```python
from build123d import *

# Parameters (mm, degrees)
F0_R      = 15.5
F1_DEPTH  = 75
F4_R      = 25.113735
F5_DEPTH  = 55.001
F6_R      = 7.557
F7_DEPTH  = 75.001
F9_DEPTH  = 35
F10_R     = 7.557
F10_R_2   = 6.35
F11_DEPTH = 35
F13_D     = 5
F13_DEPTH = 15


with BuildPart() as f1:
    # F0 (on Front) → F1 (new body)
    with BuildSketch(Plane.XZ):
        Circle(F0_R)
    extrude(amount=F1_DEPTH)

    # F2 (on Right) → F3 (revolve, cut)
    with BuildSketch(Plane.YZ):
        Polygon((-17, 12), (0, 12), (0, 15.5), (-20, 15.5), (-20, 11), (-17, 11), align=None)
    revolve(axis=Axis((0, -40.473823, 0), (0, -1, 0)), mode=Mode.SUBTRACT)

    # F4 (on face) → F5 (cut, through all)
    with BuildSketch(Plane(origin=(0, -20, 0), x_dir=(-1, 0, 0), z_dir=(0, 1, 0))):
        Circle(F4_R)
        Polygon((-13.423394, 7.75), (0, 15.5), (13.423394, 7.75), (13.423394, -7.75), (0, -15.5), (-13.423394, -7.75), align=None, mode=Mode.SUBTRACT)
    extrude(amount=-F5_DEPTH, mode=Mode.SUBTRACT)

    # F6 (on face) → F7 (cut, through all)
    with BuildSketch(Plane(origin=(0, 0, 0), x_dir=(-1, 0, 0), z_dir=(0, 1, 0))):
        Circle(F6_R)
    extrude(amount=-F7_DEPTH, mode=Mode.SUBTRACT)

    # F8 (on face) → F9 (cut)
    with BuildSketch(Plane.XZ.offset(75)):
        Polygon((-0.463436, 5.802696), (-2.763436, 9.786412), (-7.093564, 7.286412), (-4.793564, 3.302696), align=None)
    extrude(amount=-F9_DEPTH, mode=Mode.SUBTRACT)

    # F10 (on face) → F11 (join)
    with BuildSketch(Plane(origin=(0, 0, 0), x_dir=(-1, 0, 0), z_dir=(0, 1, 0))):
        Circle(F10_R)
        Circle(F10_R_2, mode=Mode.SUBTRACT)
    extrude(amount=-F11_DEPTH)

    # F13
    with Locations(Plane(origin=(-6.711697, 0, 11.625), x_dir=(0.866025, 0, 0.5), z_dir=(-0.5, 0, 0.866025))):
        with Locations((0, -57.5)):
            Hole(F13_D / 2, depth=F13_DEPTH)

    # F14 (on Right) → F15 (revolve, cut)
    with BuildSketch(Plane.YZ):
        Polygon((-20, 0), (0, 0), (0, 8.875), (-20, 6.064183), align=None)
    revolve(axis=Axis((0, -10, 0), (0, 1, 0)), mode=Mode.SUBTRACT)


solid = f1.part
```
Design review of the part built by this model. Coordinates are the model's own, in mm. A direction names the side the tool comes from. Coordinates: 2 decimals unless noted, no trailing zeros. Write each loop counter-clockwise with the first axis right and the second up, starting at its lowest first coordinate (ties: lowest second). Pieces come first, ordered by that corner, then holes. Notation, with made-up numbers: M -12.5,-35.5 L 7.5,-35.5 A9 ccw 7.5,-24.5 Z; hole C 56.5,34 d4. An arc over 180 degrees is marked long. Answer as a JSON object with one key per item and string values.
Item 1: Add section D-D, the plane y = -13. Give the boundary of the cut face in (x, z).
Outcome:
{"outline": "C 0,0 d24; hole C 0,0 d14.1"}
Item 2: Insertion check: pin 1 Ø6 at (x, y) = (8.5, -20) entering from -Z; pin 2 Ø4.5 at (x, z) = (-1.5, -2.5) entering from -Y; pin 3 Ø1 at (x, y) = (3.5, -9) entering from -Z; pin 4 Ø3 at (y, z) = (-8, 12.5) entering from +X. Each pin has a flat end and moves straight along its axis. Give the tip position at first contact, or say it passes through.
Outcome:
{"pin 1": "z = -12.32", "pin 2": "through", "pin 3": "z = -11.62", "pin 4": "x = 4.8"}
Item 3: Add section A-A, the plane z = 0. Give the boundary of the cut face in (x, y) (3 decimals), and give its area (3 significant figures).
Outcome:
{"outline": "M -13.423,-75 L -7.557,-75 L -7.557,-35 L -6.35,-35 L -6.35,-17.966 L -8.875,0 L -12,0 L -12,-17 L -11,-17 L -11,-20 L -13.423,-20 Z; M 6.35,-35 L 7.557,-35 L 7.557,-75 L 13.423,-75 L 13.423,-20 L 11,-20 L 11,-17 L 12,-17 L 12,0 L 8.875,0 L 6.35,-17.966 Z", "area": "856 mm²"}
Item 4: Add section C-C, the plane x = -5. State how many separate pieces and enclosed holes the cut face has, and give its area (3 significant figures).
Outcome:
{"separate pieces": "3", "enclosed holes": "0", "area": "908 mm²"}
Item 5: Wall thickness on probe 1 along Y at (x, z) = (9, -6.5); probe 2 along X at (y, z) = (-45.5, 0); probe 3 along X at (y, z) = (-26.5, 0): over which ranges is each line inside the solid? List them lowest first.
Outcome:
{"probe 1": "-75 to -20, -17 to 0", "probe 2": "-13.42 to -7.56, 7.56 to 13.42", "probe 3": "-13.42 to -6.35, 6.35 to 13.42"}
Item 6: Machinability: for faces 1 (the cylindrical face through (-0.53, -8.38, -11.99)), 2 (the flat face through (-11, -20, 2)), 3 (the flat face through (-13.423, -47, 0)), 4 (the flat face through (13.423, -47, 0)), 5 (the flat face through (-4.898, -61.634, 8.554)), which of the approach directions +Z, -Z, +X, -X, +Y, -Y give a long, thin tool a straight path to every point of the face, cutting with its end or side? Answer none if there is none.
Outcome:
{"face 1": "+Y", "face 2": "none", "face 3": "+Z, -Z, -X, +Y, -Y", "face 4": "+Z, -Z, +X, +Y, -Y", "face 5": "-Y"}
Item 7: Add section B-B, the plane y = -45.5. Give the boundary of the cut face in (x, z).
Outcome:
{"outline": "M -13.42,-7.75 L 0,-15.5 L 13.42,-7.75 L 13.42,7.75 L 0,15.5 L -13.42,7.75 Z; hole M -7.09,7.29 L -5.73,4.93 A7.56 ccw long -1.4,7.43 L -2.76,9.79 Z"}
Item 8: Draft analysis for pull direction Y (two halves, no side actions). For faces 6 (the cylindrical face through (1.38, -26.36, -6.2)), 7 (the cylindrical face through (10.74, -18.48, -2.38)), 8 (the flat face through (-4, -40, 7)), state which applies: pulls with the +Y half, pulls with the -Y half, needs draft (parallel to the pull), parting line crosses it, or undercut.
Outcome:
{"face 6": "needs draft", "face 7": "undercut", "face 8": "pulls with the -Y half"}
